Autodesk Inventor part; units mm, degrees
ref_plane "YZ Plane" through (0, 0, 0) normal (1, 0, 0) x (0, 1, 0)
ref_plane "XZ Plane" through (0, 0, 0) normal (0, 1, 0) x (-1, 0, 0)
ref_plane "XY Plane" through (0, 0, 0) normal (0, 0, 1) x (1, 0, 0)
sketch "Sketch1" plane through (0, 0, 0) normal (0, 0, 1) x (1, 0, 0)
  line L0 (-41.5, 5) -> (41.5, 5)
  line L1 (41.5, 5) -> (41.5, -5)
  line L2 (41.5, -5) -> (-41.5, -5)
  line L3 (-41.5, -5) -> (-41.5, 5)
  line L4 (-41.5, 5) -> (41.5, -5) construction
  line L5 (41.5, 5) -> (-41.5, -5) construction
  point P0 (0, 0)
  dimension "d0" = 83
  dimension "d1" = 10
extrude "Extrusion1" add sketch "Sketch1" along normal blind 0.4
sketch "Sketch2" plane through (0, 0, 0.4) normal (0, 0, 1) x (1, 0, 0)
  line L0 (31.2, 2.4) -> (36, 2.4)
  line L1 (36, 2.4) -> (36, -2.4)
  line L2 (36, -2.4) -> (31.2, -2.4)
  line L3 (31.2, -2.4) -> (31.2, 2.4)
  line L4 (31.2, 2.4) -> (36, -2.4) construction
  line L5 (36, 2.4) -> (31.2, -2.4) construction
  line L6 (-41.5, 5) -> (-41.5, -5)
  line L7 (41.5, -5) -> (41.5, 5)
  line L8 (14.4, 2.4) -> (19.2, 2.4)
  line L9 (19.2, 2.4) -> (19.2, -2.4)
  line L10 (19.2, -2.4) -> (14.4, -2.4)
  line L11 (14.4, -2.4) -> (14.4, 2.4)
  line L12 (14.4, 2.4) -> (19.2, -2.4) construction
  line L13 (19.2, 2.4) -> (14.4, -2.4) construction
  line L14 (-2.4, 2.4) -> (2.4, 2.4)
  line L15 (2.4, 2.4) -> (2.4, -2.4)
  line L16 (2.4, -2.4) -> (-2.4, -2.4)
  line L17 (-2.4, -2.4) -> (-2.4, 2.4)
  line L18 (-2.4, 2.4) -> (2.4, -2.4) construction
  line L19 (2.4, 2.4) -> (-2.4, -2.4) construction
  line L20 (-19.2, 2.4) -> (-14.4, 2.4)
  line L21 (-14.4, 2.4) -> (-14.4, -2.4)
  line L22 (-14.4, -2.4) -> (-19.2, -2.4)
  line L23 (-19.2, -2.4) -> (-19.2, 2.4)
  line L24 (-19.2, 2.4) -> (-14.4, -2.4) construction
  line L25 (-14.4, 2.4) -> (-19.2, -2.4) construction
  line L26 (-36, 2.4) -> (-31.2, 2.4)
  line L27 (-31.2, 2.4) -> (-31.2, -2.4)
  line L28 (-31.2, -2.4) -> (-36, -2.4)
  line L29 (-36, -2.4) -> (-36, 2.4)
  line L30 (-36, 2.4) -> (-31.2, -2.4) construction
  line L31 (-31.2, 2.4) -> (-36, -2.4) construction
  point P0 (0, 0)
  point P1 (33.6, 0)
  point P2 (33.6, 0)
  point P3 (-41.5, 0)
  point P4 (16.8, 0)
  point P5 (16.8, 0)
  point P6 (0, 0)
  point P7 (0, 0)
  point P8 (-16.8, 0)
  point P9 (-16.8, 0)
  point P10 (-33.6, 0)
  point P11 (-33.6, 0)
  dimension "d4" = 4.8
  dimension "d5" = 4.8
  dimension "d6" = 5.5
  dimension "d9" = 16.8
extrude "Extrusion2" add sketch "Sketch2" along normal blind 1.5
sketch "Sketch3" plane through (0, 0, 1.9) normal (0, 0, 1) x (1, 0, 0)
  circle A0 centre (33.6, 0) radius 2
  line L0 (36, -2.4) -> (36, 2.4)
  line L1 (36, 2.4) -> (31.2, 2.4)
  point P0 (0, 0)
  point P1 (36, 0)
  point P2 (33.6, 2.4)
  dimension "d16" = 4
extrude "Extrusion3" cut sketch "Sketch3" against normal blind 0.2
pattern_linear "Rectangular Pattern1" count 5 spacing 16.8 along (-1, 0, 0) of "Extrusion3"
properties part number "LEDStrip 5x"
Design review of the part built by this model. Coordinates are the model's own, in mm. A direction names the side the tool comes from. Round coordinates to 2 decimals unless told otherwise and drop trailing zeros. Write each loop counter-clockwise with the first axis right and the second up, starting at its lowest first coordinate (ties: lowest second). Pieces come first, ordered by that corner, then holes. Notation, with made-up numbers: M 35,12.25 L 90,12.25 A30 ccw 90,48.25 Z; hole C 78.25,40.5 d7. An arc over 180 degrees is marked long. One line per item, written item: value. Start each with the question number.
1. For faces 1 (the face through (-14.4, 0, 1)), 2 (the face through (17, 2.4, 1)), 3 (the face through (17, -2.4, 1)), list the 3-axis set-ups (+Z, -Z, +X, -X, +Y, -Y) from which the entire face can be reached by the end or side of a thin tool; tool diameter is ignored.
2. To check wall thickness, follow probe 1 along X at (y, z) = (1, 1.2); probe 2 along Y at (x, z) = (17, 1.85); probe 3 along Z at (x, y) = (38, -2). State the ranges of each line that lie inside material, in increasing order. Write a range as from..to.
3. Clearance check with flat-ended pins moving along their axes: P1, Ø0.8, axis at x = -15.5, z = 1, coming from the +Y side; P2, Ø1.5, axis at x = 6.5, y = 1, coming from the +Z side; P3, Ø0.8, axis at x = 17, z = 1, coming from the -Y side; P4, Ø1, axis at y = -3, z = 1, coming from the -X side. State where each tip first meets the part, or that it passes through.
4. Take a section at B-B on x = -16.8. State the section outline as (y, z) points, then the cut area to 3 significant figures.
5. Draft analysis for pull direction X (two halves, no side actions). For faces 4 (the face through (33.6, 2.2, 1.9)), 5 (the face through (31.2, 0, 1)), state which applies: pulls with the +X half, pulls with the -X half, needs draft (parallel to the pull), parting line crosses it, or undercut.
6. Take a section at D-D on x = -33. State the section outline as (y, z) points.
7. Take a section at C-C on y = 4. State the section outline as (x, z) points.
8. Take a section at A-A on z = 1.25. State the section outline as (x, y) points, then the cut area to 3 significant figures.
Computed:
1. face 1: +Z, +Y, -Y
1. face 2: +Z, +X, -X, +Y
1. face 3: +Z, +X, -X, -Y
2. probe 1: x = -36..-31.2, -19.2..-14.4, -2.4..2.4, 14.4..19.2, 31.2..36
2. probe 2: y = -2.4..-1.99, 1.99..2.4
2. probe 3: z = 0..0.4
3. P1: stops at y = 2.4
3. P2: stops at z = 0.4
3. P3: stops at y = -2.4
3. P4: passes through
4. outline: M -5,0 L 5,0 L 5,0.4 L 2.4,0.4 L 2.4,1.9 L 2,1.9 L 2,1.7 L -2,1.7 L -2,1.9 L -2.4,1.9 L -2.4,0.4 L -5,0.4 Z
4. area: 10.4 mm²
5. face 4: needs draft
5. face 5: undercut
6. outline: M -5,0 L 5,0 L 5,0.4 L 2.4,0.4 L 2.4,1.9 L 1.91,1.9 L 1.91,1.7 L -1.91,1.7 L -1.91,1.9 L -2.4,1.9 L -2.4,0.4 L -5,0.4 Z
7. outline: M -41.5,0 L 41.5,0 L 41.5,0.4 L -41.5,0.4 Z
8. outline: M -36,-2.4 L -31.2,-2.4 L -31.2,2.4 L -36,2.4 Z; M -19.2,-2.4 L -14.4,-2.4 L -14.4,2.4 L -19.2,2.4 Z; M -2.4,-2.4 L 2.4,-2.4 L 2.4,2.4 L -2.4,2.4 Z; M 14.4,-2.4 L 19.2,-2.4 L 19.2,2.4 L 14.4,2.4 Z; M 31.2,-2.4 L 36,-2.4 L 36,2.4 L 31.2,2.4 Z
8. area: 115 mm²
